Source: CAD feature listing. Evaluate the final solid. Frame: model axes, mm. A direction names the side the tool comes from. Coordinates: 2 decimals unless noted, no trailing zeros. Loops run counter-clockwise (first coordinate to the right, second up) from the corner with the lowest first, then second, coordinate; pieces in that order, holes last. Notation, with made-up numbers: (-11.75, 14.5) -> (-3.75, 14.5) arc R17 ccw to (-3.75, 41.5) -> close; hole circle Ø4 at (80.25, -35). An arc over 180 degrees is marked (long way). Answer as CSV lines item,"result".
from build123d import *

# Parameters (mm, degrees)
SKETCH_1_R              = 9.5
EXTRUDE_1_DEPTH         = 1
SKETCH_2_R              = 7.83
EXTRUDE_2_DEPTH         = 11
SKETCH_3_R              = 9.5
EXTRUDE_3_DEPTH         = 1
SKETCH_4_R              = 6
EXTRUDE_4_DEPTH         = 10
SKETCH_5_R              = 2.5
CUT_EXTRUDE_1_DEPTH     = 27.636441204
HOLE_WIZARD_M4_1_REACH  = 28.281
HOLE_WIZARD_M4_1_BORE_R = 1.65
HOLE_WIZARD_M4_2_REACH  = 28.348
HOLE_WIZARD_M4_2_BORE_R = 1.65


with BuildPart() as part:
    # 草图1 → 凸台-拉伸1 (new body)
    with BuildSketch(Plane(origin=(0, 0, 0), x_dir=(1, 0, 0), z_dir=(0, 1, 0))):
        with Locations(Location((0, 0, 0), (0, 0, 270))):
            Circle(SKETCH_1_R)
    extrude(amount=EXTRUDE_1_DEPTH)

    # 草图2 → 凸台-拉伸2 (add)
    with BuildSketch(Plane(origin=(0, 1, 0), x_dir=(1, 0, 0), z_dir=(0, 1, 0))):
        with Locations(Location((0, 0, 0), (0, 0, 270))):
            Circle(SKETCH_2_R)
    extrude(amount=EXTRUDE_2_DEPTH)

    # 草图3 → 凸台-拉伸3 (add)
    with BuildSketch(Plane(origin=(0, 12, 0), x_dir=(1, 0, 0), z_dir=(0, 1, 0))):
        with Locations(Location((0, 0, 0), (0, 0, 270))):
            Circle(SKETCH_3_R)
    extrude(amount=EXTRUDE_3_DEPTH)

    # 草图4 → 凸台-拉伸4 (add)
    with BuildSketch(Plane(origin=(0, 13, 0), x_dir=(1, 0, 0), z_dir=(0, 1, 0))):
        with Locations(Location((0, 0, 0), (0, 0, 270))):
            Circle(SKETCH_4_R)
    extrude(amount=EXTRUDE_4_DEPTH)

    # 草图5 → 切除-拉伸1 (cut, through all)
    with BuildSketch(Plane(origin=(0, 23, 0), x_dir=(1, 0, 0), z_dir=(0, 1, 0))):
        with Locations(Location((0, 0, 0), (0, 0, 270))):
            Circle(SKETCH_5_R)
    extrude(amount=-CUT_EXTRUDE_1_DEPTH, mode=Mode.SUBTRACT)

    # M4 螺纹孔1 bore (on position points) → M4 螺纹孔1 (cut, up to next)
    with BuildSketch(Plane(origin=(-5.992739495, 18.833476166, -0.295081925), x_dir=(0.04918032089, 0, -0.998789915867), z_dir=(-0.998789915867, 0, -0.04918032089)), mode=Mode.PRIVATE) as hole_wizard_m4_1_sk1:
        Circle(HOLE_WIZARD_M4_1_BORE_R)
    hole_wizard_m4_1_tool1 = extrude(hole_wizard_m4_1_sk1.sketch, amount=-HOLE_WIZARD_M4_1_REACH, mode=Mode.PRIVATE) & part.part
    add(hole_wizard_m4_1_tool1.solids().sort_by_distance((-5.992739, 18.833476, -0.295082))[0], mode=Mode.SUBTRACT)

    # M4 螺纹孔2 bore (on position points) → M4 螺纹孔2 (cut, up to next)
    with BuildSketch(Plane(origin=(0.168248466, 18.988782442, -5.997640574), x_dir=(-0.999606762316, 0, -0.028041411034), z_dir=(0.028041411034, 0, -0.999606762316)), mode=Mode.PRIVATE) as hole_wizard_m4_2_sk1:
        Circle(HOLE_WIZARD_M4_2_BORE_R)
    hole_wizard_m4_2_tool1 = extrude(hole_wizard_m4_2_sk1.sketch, amount=-HOLE_WIZARD_M4_2_REACH, mode=Mode.PRIVATE) & part.part
    add(hole_wizard_m4_2_tool1.solids().sort_by_distance((0.168248, 18.988782, -5.997641))[0], mode=Mode.SUBTRACT)


solid = part.part
(1) Material intervals for L1, parallel to Y at x = -8.5, z = 3.25; L2, parallel to Y at x = -5.25, z = -0.25; L3, parallel to Y at x = 2.25, z = 6.75, sorted ascending. Write a range as [from, to].
Computed values:
L1,"[0, 1], [12, 13]"
L2,"[0, 17.18], [20.48, 23]"
L3,"[0, 13]"
(2) Draft query along X for faces 4 (the cylindrical face through (-4.764, 6.423, -6.214)), 5 (the cylindrical face through (0.47, 17.38, -3.96)), 6 (the cylindrical face through (-3.981, 20.444, 0.162)), 7 (the flat face through (-2, 0, 2)). Return one class per face: released by +X, released by -X, zero draft, split by the parting line, or undercut.
Computed values:
face 4,"split by the parting line"
face 5,"undercut"
face 6,"undercut"
face 7,"zero draft"
(3) Access query for faces 1 (the flat face through (-6.2, 13, -0.1)), 2 (the flat face through (8, 12, 1)), 3 (the cylindrical face through (-5.78, 12.49, -7.54)). Directions: +Z, -Z, +X, -X, +Y, -Y. A direction counts if a zero-diameter tool reaches every point of the face in a straight line with its end or side. Return the directions, or none.
Computed values:
face 1,"+Y"
face 2,"none"
face 3,"+Y, -Y"
(4) Cut plane B-B (x = -6.5). Return the cut outline in (y, z), then the cut area to 3 significant figures.
Computed values:
outline,"(0, -6.93) -> (1, -6.93) -> (1, -4.37) -> (12, -4.37) -> (12, -6.93) -> (13, -6.93) -> (13, 6.93) -> (12, 6.93) -> (12, 4.37) -> (1, 4.37) -> (1, 6.93) -> (0, 6.93) -> close"
area,"124 mm^2"
(5) Cut plane A-A (y = 14.5). Return the cut outline in (x, z), then the cut area to 3 significant figures.
Computed values:
outline,"circle Ø12 at (0, 0); hole circle Ø5 at (0, 0)"
area,"93.5 mm^2"
(6) Cut plane C-C (z = 5.5). Return the cut outline in (x, y), then the cut area to 3 significant figures.
Computed values:
outline,"(-7.75, 0) -> (7.75, 0) -> (7.75, 1) -> (5.57, 1) -> (5.57, 12) -> (7.75, 12) -> (7.75, 13) -> (2.4, 13) -> (2.4, 23) -> (-2.4, 23) -> (-2.4, 13) -> (-7.75, 13) -> (-7.75, 12) -> (-5.57, 12) -> (-5.57, 1) -> (-7.75, 1) -> close"
area,"202 mm^2"
(7) Cut plane D-D (y = 5.25). Return the cut outline in (x, z).
Computed values:
outline,"circle Ø15.66 at (0, 0); hole circle Ø5 at (0, 0)"
(8) Pin query (flat end, axial travel): pin 1 Ø1.5 at (y, z) = (13, 2) entering from +X; pin 2 Ø1 at (y, z) = (14.5, 1) entering from +X; pin 3 Ø4 at (x, y) = (-7.5, 16) entering from +Z; pin 4 Ø4.5 at (x, z) = (0, 0) entering from -Y. Return the tip coordinate at first contact, or that it passes through.
Computed values:
pin 1,"x = 9.42"
pin 2,"x = 5.98"
pin 3,"z = 2.4"
pin 4,"through"
